```python
from build123d import *
from OCP.BRepFilletAPI import BRepFilletAPI_MakeFillet

# Parameters (mm, degrees)
SCHIZZO2_R                   = 1.575
SCHIZZO2_R_2                 = 1.525
ESTRUSIONE_ESTRUSIONE1_DEPTH = 1.5
RACCORDO1_R1                 = 3
RACCORDO1_R2                 = 10
SCHIZZO4_R                   = 1.55
ESTRUSIONE_ESTRUSIONE2_DEPTH = 2.5
ESTRUSIONE_ESTRUSIONE3_DEPTH = 2.5


with BuildPart() as part:
    # Schizzo2 → Estrusione-Estrusione1 (new body)
    with BuildSketch(Plane.XY):
        Polygon((10.835450111, 45.456844872), (10.835450111, 104.878132603), (-7.726239407, 141.30749945), (4.747851932, 147.663366447), (24.835450111, 108.23923523), (24.835450111, 45.456844872), align=None)
        with Locations((17.835450111, 52.456844872)):
            Circle(SCHIZZO2_R, mode=Mode.SUBTRACT)
        with Locations((1.688739761, 138.248387279)):
            Circle(SCHIZZO2_R_2, mode=Mode.SUBTRACT)
        with Locations((7.590616257, 126.665302465)):
            Circle(SCHIZZO2_R_2, mode=Mode.SUBTRACT)
    extrude(amount=ESTRUSIONE_ESTRUSIONE1_DEPTH)

    # Raccordo1: one fillet with a radius per group of edges: ONE call of the kernel's fillet builder (fillet() takes one radius for all edges)
    raccordo1_edges_1 = [part.edges().sort_by_distance(p)[0] for p in [
        (4.747851932, 147.663366447, 0.75),
        (-7.726239407, 141.30749945, 0.75),
        (10.835450111, 45.456844872, 0.75),
        (24.835450111, 45.456844872, 0.75),
    ]]
    raccordo1_edges_2 = [part.edges().sort_by_distance(p)[0] for p in [
        (24.835450111, 108.23923523, 0.75),
        (10.835450111, 104.878132603, 0.75),
    ]]
    raccordo1 = BRepFilletAPI_MakeFillet(part.part.solid().wrapped)
    for e in raccordo1_edges_1:
        raccordo1.Add(RACCORDO1_R1, e.wrapped)
    for e in raccordo1_edges_2:
        raccordo1.Add(RACCORDO1_R2, e.wrapped)
    add(Compound.cast(raccordo1.Shape()), mode=Mode.REPLACE)

    # Schizzo4 → Estrusione-Estrusione2 (add)
    with BuildSketch(Plane(origin=(0, 0, 0), x_dir=(-1, 0, 0), z_dir=(0, 0, -1))):
        with Locations(Location((-13.532140626, 53.421016786, 0), (0, 0, 180))):
            Circle(SCHIZZO4_R)
        with Locations(Location((-22.138759596, 51.492672958, 0), (0, 0, 180))):
            Circle(SCHIZZO4_R)
    extrude(amount=ESTRUSIONE_ESTRUSIONE2_DEPTH)

    # Schizzo5 → Estrusione-Estrusione3 (add)
    with BuildSketch(Plane(origin=(0, 0, 0), x_dir=(-1, 0, 0), z_dir=(0, 0, -1))):
        with BuildLine():
            Line((-24.835450111, 63.770542244), (-19.320054404, 59.217112451))
            Line((-19.320054404, 59.217112451), (-14.402001203, 59.217112451))
            add(Edge.make_bspline(
                [(-14.402001203, 59.217112451), (-13.28177849, 59.164141407), (-11.913165696, 58.833942628), (-10.835450111, 58.162340852)],
                knots=[0, 0, 0, 0, 0.33692331, 0.33692331, 0.33692331, 0.33692331], degree=3))
            Line((-10.835450111, 58.162340852), (-10.835450111, 102.477345012))
            ThreePointArc((-10.835450111, 102.477345012), (-10.559149315, 104.811798651), (-9.745515353, 107.01725001))
            Line((-9.745515353, 107.01725001), (-6.567581855, 113.254295679))
            Line((-6.567581855, 113.254295679), (-8.349594903, 114.162276678))
            Line((-8.349594903, 114.162276678), (-11.527528401, 107.925231009))
            ThreePointArc((-11.527528401, 107.925231009), (-12.503889156, 105.278689378), (-12.835450111, 102.477345012))
            Line((-12.835450111, 102.477345012), (-12.835450111, 69.217112451))
            Line((-12.835450111, 69.217112451), (-22.835450111, 69.217112451))
            Line((-22.835450111, 69.217112451), (-22.835450111, 105.838447639))
            ThreePointArc((-22.835450111, 105.838447639), (-22.614409474, 107.70601055), (-21.963502304, 109.470371637))
            Line((-21.963502304, 109.470371637), (-17.259660145, 118.702181676))
            Line((-17.259660145, 118.702181676), (-19.041673193, 119.610162675))
            Line((-19.041673193, 119.610162675), (-23.745515353, 110.378352637))
            ThreePointArc((-23.745515353, 110.378352637), (-24.559149315, 108.172901278), (-24.835450111, 105.838447639))
            Line((-24.835450111, 105.838447639), (-24.835450111, 63.770542244))
        make_face()
        with BuildLine():
            Line((-19.320054404, 59.217112451), (-24.835450111, 63.770542244))
            ThreePointArc((-24.835450111, 63.770542244), (-24.711960876, 63.245404245), (-24.488566128, 62.75437034))
            ThreePointArc((-24.488566128, 62.75437034), (-22.305073607, 60.400160674), (-19.320054404, 59.217112451))
        make_face()
    extrude(amount=ESTRUSIONE_ESTRUSIONE3_DEPTH)


solid = part.part
```
Input: part model. Units: mm. Frame: model coordinates. A direction names the side the tool comes from. Give positions to 0.01 mm unless a question says otherwise; leave off trailing zeros. Order: outer loops, then holes, each group sorted by start corner. A loop starts at its lowest first (then second) coordinate and runs counter-clockwise, first axis right, second up. Notation, with made-up numbers: M 49.5,-23.5 L 107.5,-23.5 A15 cw 107.5,-1.5 Z; hole C 11.25,-26.75 d1. An arc over 180 degrees is marked long. Return JSON: item names as keys, results as strings.
Item 1: First-contact query: P1, Ø2, axis at y = 100, z = -1.5, coming from the -X side; P2, Ø12, axis at x = 9, y = 60.5, coming from the -Z side; P3, Ø2, axis at x = 19.5, z = -1.5, coming from the +Y side; P4, Ø4, axis at x = 7.59, y = 126.67, coming from the -Z side. Flat tips, straight axial feed; report the tip coordinate or a pass-through.
Solutions:
{"P1": "x = 10.84", "P2": "z = -2.5", "P3": "y = 119.61", "P4": "z = 0"}
Item 2: Cut plane A-A (z = -1.1). State how many separate pieces and enclosed holes the cut face has, then the cut area to 3 significant figures.
Solutions:
{"separate pieces": "3", "enclosed holes": "0", "area": "342 mm^2"}
Item 3: Ray query, probe 1 along Y at (x, z) = (22, -1.4); probe 2 along X at (y, z) = (72.5, -0.9); probe 3 along Z at (x, y) = (2, 128). Return the intervals inside material, ascending.
Solutions:
{"probe 1": "49.95 to 53.04, 60.2 to 69.22, 109.4 to 113.8", "probe 2": "10.84 to 12.84, 22.84 to 24.84", "probe 3": "0 to 1.5"}
Item 4: Cut plane B-B (y = 60.5). Return loops of the section in (x, z).
Solutions:
{"outline": "M 10.84,-2.5 L 22.45,-2.5 L 22.45,0 L 24.84,0 L 24.84,1.5 L 10.84,1.5 Z"}
Item 5: Cut plane C-C (x = -3). Return loops of the section in (y, z), then the cut area to 3 significant figures.
Solutions:
{"outline": "M 132.03,0 L 143.72,0 L 143.72,1.5 L 132.03,1.5 Z", "area": "17.5 mm^2"}
Item 6: Pull-direction query (X, two-part tool) for faces 6 (the cylindrical face through (-6.554, 140.892, 0.76)), 7 (the cylindrical face through (21.937, 49.956, -1.232)), 8 (the flat face through (17, 59.217, -1)), 9 (the cylindrical face through (13.33, 51.884, -1.232)); classes: +X half, -X half, draft (parallel to the pull), parting line (faces both ways), or undercut.
Solutions:
{"face 6": "-X half", "face 7": "undercut", "face 8": "draft", "face 9": "undercut"}
Item 7: Access query for faces 1 (the flat face through (18, 55, 0)), 2 (the flat face through (7.446, 113.702, -1.232)), 3 (the cylindrical face through (11.69, 46.36, 0.76)), 4 (the flat face through (12.835, 86, -1)), 5 (the cylindrical face through (22.342, 60.426, -1.232)). Directions: +Z, -Z, +X, -X, +Y, -Y. A direction counts if a zero-diameter tool reaches every point of the face in a straight line with its end or side. Return the directions, or none.
Solutions:
{"face 1": "-Z", "face 2": "-Z, -X, +Y", "face 3": "+Z, -Z, -X, -Y", "face 4": "-Z, +Y", "face 5": "-Z, +X"}
Item 8: Cut plane D-D (y = 121). Return loops of the section in (x, z), then the cut area to 3 significant figures.
Solutions:
{"outline": "M 2.62,0 L 18.33,0 L 18.33,1.5 L 2.62,1.5 Z", "area": "23.6 mm^2"}
